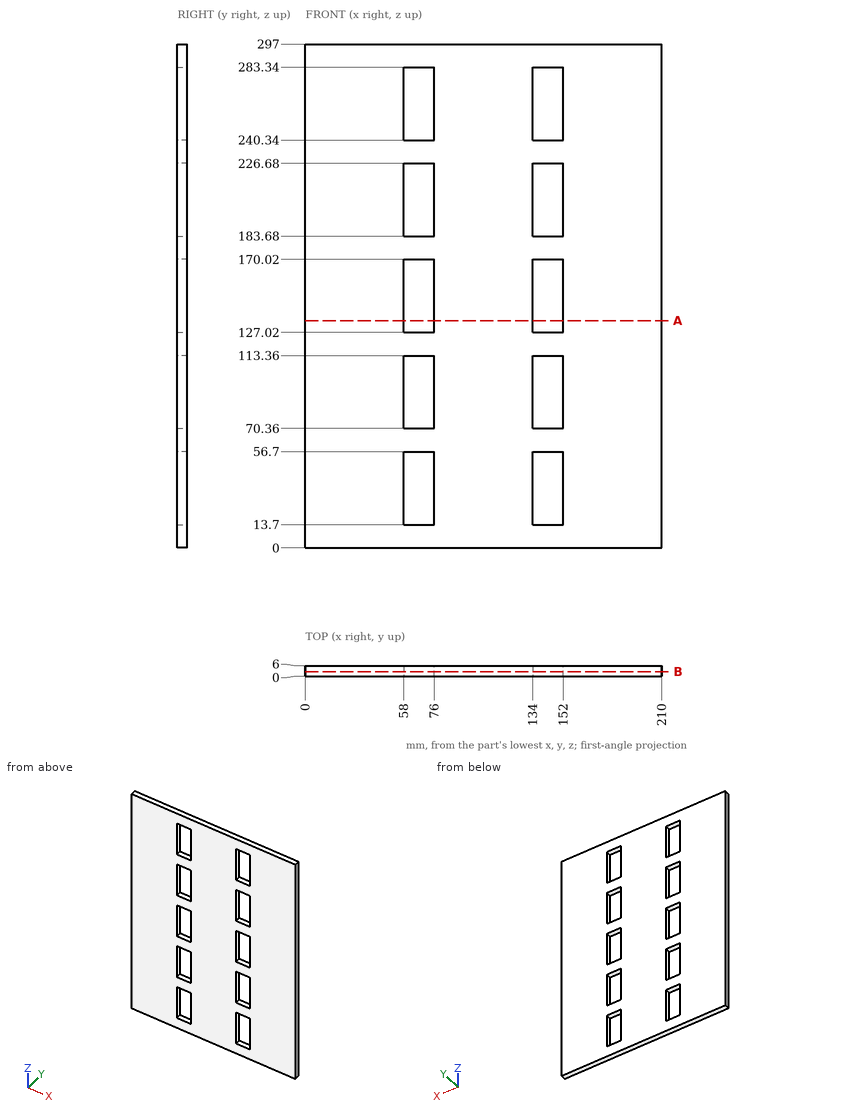
Part print with two shaded views. Sizes in mm from the minimum x, y, z corner. Round coordinates to 2 decimals unless told otherwise and drop trailing zeros. Write each loop counter-clockwise with the first axis right and the second up, starting at its lowest first coordinate (ties: lowest second). Pieces come first, ordered by that corner, then holes. Notation, with made-up numbers: M 42.25,-12 L 79.25,-12 A12 ccw 79.25,7 Z; hole C -22.75,20 d4. An arc over 180 degrees is marked long. Put each result on its own line as item: value. Start each with the question number.
1) Saw through at A-A, the plane z = 134. Write the cut outline in (x, y).
2) Saw through at B-B, the plane y = 2.65. Count the separate pieces of the cut face and the enclosed holes in it, and give its area (3 significant figures).
3) Drill centre lines: probe 1 along X at (y, z) = (4.2, 53); probe 2 along Z at (x, y) = (73, 2). Where is each one in solid material? Low to high. Write a range as [from, to].
Resolved:
1. outline: M 0,0 L 58,0 L 58,6 L 0,6 Z; M 76,0 L 134,0 L 134,6 L 76,6 Z; M 152,0 L 210,0 L 210,6 L 152,6 Z
2. separate pieces: 1
2. enclosed holes: 10
2. area: 54,600 mm²
3. probe 1: [0, 58], [76, 134], [152, 210]
3. probe 2: [0, 13.7], [56.7, 70.36], [113.36, 127.02], [170.02, 183.68], [226.68, 240.34], [283.34, 297]
